Part model, mm, in its own coordinate system. Round coordinates to 2 decimals unless told otherwise and drop trailing zeros. Write each loop counter-clockwise with the first axis right and the second up, starting at its lowest first coordinate (ties: lowest second). Pieces come first, ordered by that corner, then holes.
```python
from build123d import *

# Parameters (mm, degrees)
ESQUISSE1_W        = 27
ESQUISSE1_H        = 27
ESQUISSE1_W_2      = 5
ESQUISSE1_H_2      = 5
ESQUISSE1_W_3      = 10
ESQUISSE1_H_3      = 9.5
BOSS_EXTRU_1_DEPTH = 5
CONG_1_R           = 2


with BuildPart() as part:
    # Esquisse1 → Boss.-Extru.1 (new body)
    with BuildSketch(Plane.XY):
        Polygon((0, 0), (7.5, 0), (7.5, -5), (12.5, -5), (12.5, 0), (58.5, 0), (58.5, -5), (63.5, -5), (63.5, 0), (71, 0), (71, 7.5), (76, 7.5), (76, 12.5), (71, 12.5), (71, 17.9), (38.8, 17.9), (38.8, 50), (-10, 50), (-10, 15), (-30, 15), (-30, 0), (-25, 0), (-25, -5), (-20, -5), (-20, 0), (-17, 0), (-17, 3), (-18.5, 3), (-18.5, 6), (-17, 6), (-17, 10), (-13, 10), (-13, 6), (-11.5, 6), (-11.5, 3), (-13, 3), (-13, 0), (-10, 0), (-10, -5), (-5, -5), (-5, 0), align=None)
        with Locations((20.5, 27.5)):
            Rectangle(ESQUISSE1_W, ESQUISSE1_H, mode=Mode.SUBTRACT)
        with Locations((-2.5, 40)):
            Rectangle(ESQUISSE1_W_2, ESQUISSE1_H_2, mode=Mode.SUBTRACT)
        with Locations((-2.5, 10)):
            Rectangle(ESQUISSE1_W_2, ESQUISSE1_H_2, mode=Mode.SUBTRACT)
        with Locations((54.45, 11.65)):
            Rectangle(ESQUISSE1_W_3, ESQUISSE1_H_3, mode=Mode.SUBTRACT)
    extrude(amount=BOSS_EXTRU_1_DEPTH)

    # Congé1
    cong_1_edges = [part.edges().sort_by_distance(p)[0] for p in [
        (7, 41, 2.5),
        (7, 14, 2.5),
        (34, 14, 2.5),
        (34, 41, 2.5),
        (49.45, 16.4, 2.5),
        (49.45, 6.9, 2.5),
        (59.45, 6.9, 2.5),
        (59.45, 16.4, 2.5),
        (-30, 0, 2.5),
        (-30, 15, 2.5),
        (-10, 15, 2.5),
        (-10, 50, 2.5),
        (38.8, 50, 2.5),
        (38.8, 17.9, 2.5),
        (71, 17.9, 2.5),
        (71, 0, 2.5),
    ]]
    fillet(cong_1_edges, radius=CONG_1_R)


solid = part.part
```
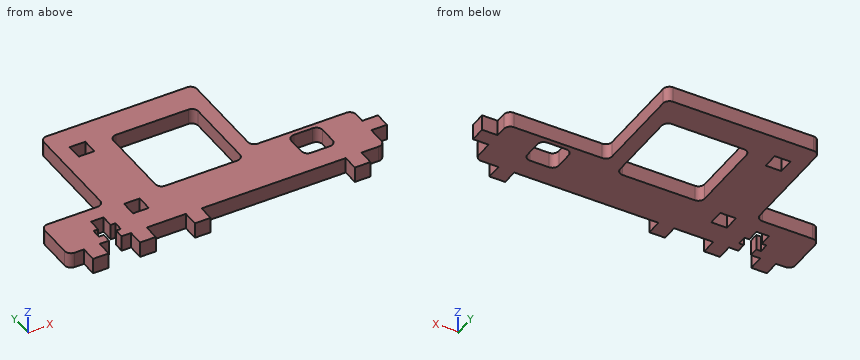
Q1. Cut at A-A on y = 4. Write the cut outline in (x, z).
Values follow:
outline: (-30, 0) - (-18.5, 0) - (-18.5, 5) - (-30, 5) - close; (-11.5, 0) - (71, 0) - (71, 5) - (-11.5, 5) - close
Q2. Cut at D-D on z = 1.8. State how many separate pieces and enclosed holes the cut face has, plus the area to 3 significant figures.
Values follow:
separate pieces: 1
enclosed holes: 4
area: 2,520 mm2
Q3. Wall check: L1, parallel to Y at x = -3, z = 3.25; L2, parallel to X at y = 38, z = 1.1; L3, parallel to X at y = 19, z = 3.3. Give the ranges that are in metal, low to high.
Values follow:
L1: y = 0 to 7.5, 12.5 to 37.5, 42.5 to 50
L2: x = -10 to -5, 0 to 7, 34 to 38.8
L3: x = -10 to 7, 34 to 39.01
Q4. Cut at B-B on x = -4. Write the cut outline in (y, z).
Values follow:
outline: (0, 0) - (7.5, 0) - (7.5, 5) - (0, 5) - close; (12.5, 0) - (37.5, 0) - (37.5, 5) - (12.5, 5) - close; (42.5, 0) - (50, 0) - (50, 5) - (42.5, 5) - close
Q5. Drop flat-ended pins along their axis: pin 1 (2.5 mm diameter, centred on y = 40.5, z = 3.5, fed in from -X); pin 2 (2.5 mm diameter, centred on x = -26.5, z = 3.5, fed in from -Y); pin 3 (3 mm diameter, centred on y = 25, z = 2.5, fed in from +X). Give the stop position or say it passes through.
Values follow:
pin 1: stops at x = -10
pin 2: stops at y = 0
pin 3: stops at x = 38.8
Q6. Cut at C-C on x = 54. Write the cut outline in (y, z), plus the area to 3 significant figures.
Values follow:
outline: (0, 0) - (6.9, 0) - (6.9, 5) - (0, 5) - close; (16.4, 0) - (17.9, 0) - (17.9, 5) - (16.4, 5) - close
area: 42.0 mm2
